```python
from build123d import *

# Parameters (mm, degrees)
SKETCH1_R           = 1.65
BOSS_EXTRUDE1_DEPTH = 1.9


with BuildPart() as part:
    # Sketch1 → Boss-Extrude1 (new body)
    with BuildSketch(Plane(origin=(0, 0, 0), x_dir=(1, 0, 0), z_dir=(0, 1, 0))):
        Polygon((-30.5, 18.5), (30.5, 18.5), (37.5, 18.5), (37.5, -18.5), (30.5, -18.5), (-30.5, -18.5), (-30.5, -5), (-50.5, -5), (-50.5, 5), (-30.5, 5), align=None)
        with Locations(Location((-26.5, 14.5, 0), (0, 0, 90))):
            Circle(SKETCH1_R, mode=Mode.SUBTRACT)
        with Locations(Location((26.5, 14.5, 0), (0, 0, 90))):
            Circle(SKETCH1_R, mode=Mode.SUBTRACT)
        with Locations(Location((26.5, -14.5, 0), (0, 0, 90))):
            Circle(SKETCH1_R, mode=Mode.SUBTRACT)
        with Locations(Location((-26.5, -14.5, 0), (0, 0, 90))):
            Circle(SKETCH1_R, mode=Mode.SUBTRACT)
    extrude(amount=BOSS_EXTRUDE1_DEPTH)


solid = part.part
```
Geometry check sheet. Reference: the model listing, model coordinates, mm. A direction names the side the tool comes from. Coordinates: 2 decimals unless noted, no trailing zeros. Loops run counter-clockwise (first coordinate to the right, second up) from the corner with the lowest first, then second, coordinate; pieces in that order, holes last.
Item 1: Sectioned sample at D-D, the plane z = 10.5. Record the boundary of the cut face in (x, y), then the cut area to 3 significant figures.
Item 2: Thickness scan on line 1 (Z direction, x = -26.5, y = 1.45); line 2 (X direction, y = 0.55, z = -14.5); line 3 (X direction, y = 1.5, z = 16). Record the ranges inside material, lowest first.
Item 3: Sectioned sample at B-B, the plane z = -14.5. Record the boundary of the cut face in (x, y).
Item 4: Sectioned sample at A-A, the plane y = 1.1. Record the boundary of the cut face in (x, z), then the cut area to 3 significant figures.
Item 5: Access from +Z, -Z, +X, -X, +Y, -Y to the whole of each face (thin tool, end or side, straight path). Record for faces 1 (the face through (-27.89, 0.94, -15.39)), 2 (the face through (-30.5, 1, -12)), 3 (the face through (-40, 1, 5)).
Item 6: Go/stop test with flat-tipped pins: pin 1 Ø0.6 at (y, z) = (0.5, 10.5) entering from -X; pin 2 Ø5.5 at (x, z) = (-26.5, -14.5) entering from -Y; pin 3 Ø1 at (x, y) = (-33, 1.5) entering from +Z. Record where each tip stops, or that it passes through.
Item 7: Release check for a two-part mould opening along X. For faces 4 (the face through (25.11, 0.94, -15.39)), 5 (the face through (-27.89, 0.94, 13.61)), 6 (the face through (4, 0, 0)), 7 (the face through (-30.5, 1, 12)) record: released by +X, released by -X, zero draft, split by the parting line, or undercut.
Item 8: Sectioned sample at C-C, the plane x = -26.5. Record the boundary of the cut face in (y, z), then the cut area to 3 significant figures.
Check result:
1. outline: (-30.5, 0) - (37.5, 0) - (37.5, 1.9) - (-30.5, 1.9) - close
1. area: 129 mm2
2. line 1: z = -18.5 to -16.15, -12.85 to 12.85, 16.15 to 18.5
2. line 2: x = -30.5 to -28.15, -24.85 to 24.85, 28.15 to 37.5
2. line 3: x = -30.5 to -27.19, -25.81 to 25.81, 27.19 to 37.5
3. outline: (-30.5, 0) - (-28.15, 0) - (-28.15, 1.9) - (-30.5, 1.9) - close; (-24.85, 0) - (24.85, 0) - (24.85, 1.9) - (-24.85, 1.9) - close; (28.15, 0) - (37.5, 0) - (37.5, 1.9) - (28.15, 1.9) - close
4. outline: (-50.5, -5) - (-30.5, -5) - (-30.5, -18.5) - (37.5, -18.5) - (37.5, 18.5) - (-30.5, 18.5) - (-30.5, 5) - (-50.5, 5) - close; hole circle Ø3.3 at (-26.5, -14.5); hole circle Ø3.3 at (-26.5, 14.5); hole circle Ø3.3 at (26.5, -14.5); hole circle Ø3.3 at (26.5, 14.5)
4. area: 2,680 mm2
5. face 1: +Y, -Y
5. face 2: -Z, -X, +Y, -Y
5. face 3: +Z, -X, +Y, -Y
6. pin 1: stops at x = -30.5
6. pin 2: stops at y = 0
6. pin 3: stops at z = 5
7. face 4: undercut
7. face 5: undercut
7. face 6: zero draft
7. face 7: released by -X
8. outline: (0, -18.5) - (1.9, -18.5) - (1.9, -16.15) - (0, -16.15) - close; (0, -12.85) - (1.9, -12.85) - (1.9, 12.85) - (0, 12.85) - close; (0, 16.15) - (1.9, 16.15) - (1.9, 18.5) - (0, 18.5) - close
8. area: 57.8 mm2
